Input: dimensioned drawing with shaded views. Units: mm. Origin: part minimum x, y, z. A direction names the side the tool comes from. Give positions to 0.01 mm unless a question says otherwise; leave off trailing zeros. Order: outer loops, then holes, each group sorted by start corner. A loop starts at its lowest first (then second) coordinate and runs counter-clockwise, first axis right, second up. Notation, with made-up numbers: (11.5, 33.5) - (18.5, 33.5) arc R19 cw to (18.5, 42.5) - close; hole circle Ø8 at (-37, 64.5). An arc over 180 degrees is marked (long way). Use a Markdown table: item, result.
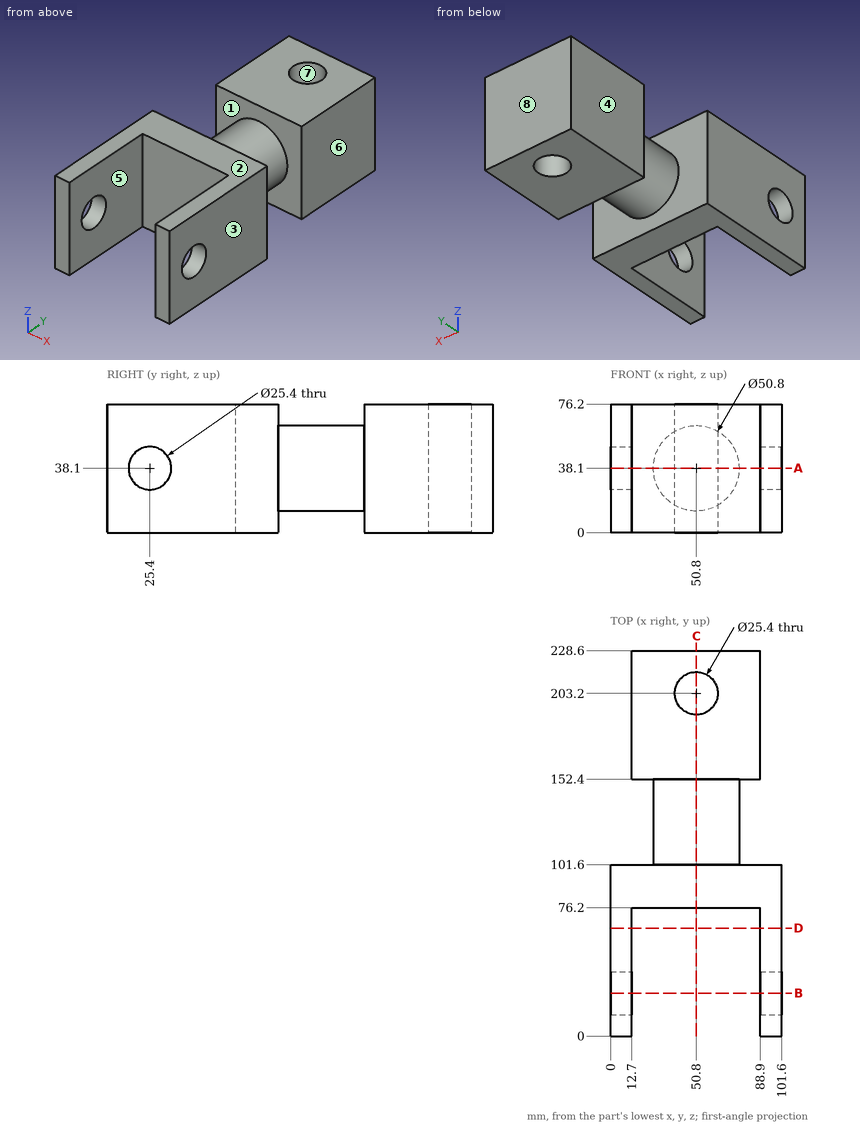
1. Mould query, pull axis X, two halves, no side actions, for the marked faces 6, 7 and 8. Classes: pulls with the +X half, pulls with the -X half, needs draft (parallel to the pull), parting line crosses it, or undercut.
Response:
| item | result |
|---|---|
| face 6 | pulls with the +X half |
| face 7 | undercut |
| face 8 | needs draft |
2. Pin query (flat end, axial travel): pin 1 (5 mm diameter, centred on y = 189.5, z = 42, fed in from -X); pin 2 (4 mm diameter, centred on x = 78.5, z = 17, fed in from -Y); pin 3 (1 mm diameter, centred on y = 176.5, z = 63, fed in from +X). Return the tip coordinate at first contact, or that it passes through.
Response:
| item | result |
|---|---|
| pin 1 | stops at x = 12.7 |
| pin 2 | stops at y = 76.2 |
| pin 3 | stops at x = 88.9 |
3. Section query C-C (x = 50.8). Return loops of the section in (y, z), then the cut area to 3 significant figures.
Response:
| item | result |
|---|---|
| outline | (76.2, 0) - (101.6, 0) - (101.6, 12.7) - (152.4, 12.7) - (152.4, 0) - (190.5, 0) - (190.5, 76.2) - (152.4, 76.2) - (152.4, 63.5) - (101.6, 63.5) - (101.6, 76.2) - (76.2, 76.2) - close; (215.9, 0) - (228.6, 0) - (228.6, 76.2) - (215.9, 76.2) - close |
| area | 8,390 mm^2 |
4. Set-up query: the marked faces 1, 2, 3, 4 and 5. Return all of +Z, -Z, +X, -X, +Y, -Y with unobstructed straight access to the full face (end or side cutting, diameter ignored); none if empty.
Response:
| item | result |
|---|---|
| face 1 | none |
| face 2 | +Z, +X, -X, +Y, -Y |
| face 3 | +Z, -Z, +X, +Y, -Y |
| face 4 | +Z, -Z, -X, +Y |
| face 5 | +Z, -Z, -Y |
5. Material intervals for line 1 along Y through (x, z) = (74.5, 15.5); line 2 along X through (y, z) = (21, 4); line 3 along Y through (x, z) = (50.8, 60), sorted ascending.
Response:
| item | result |
|---|---|
| line 1 | y = 76.2 to 101.6, 152.4 to 228.6 |
| line 2 | x = 0 to 12.7, 88.9 to 101.6 |
| line 3 | y = 76.2 to 190.5, 215.9 to 228.6 |
6. Section query A-A (z = 38.1). Return loops of the section in (x, y).
Response:
| item | result |
|---|---|
| outline | (0, 0) - (12.7, 0) - (12.7, 12.7) - (0, 12.7) - close; (0, 38.1) - (12.7, 38.1) - (12.7, 76.2) - (88.9, 76.2) - (88.9, 38.1) - (101.6, 38.1) - (101.6, 101.6) - (76.2, 101.6) - (76.2, 152.4) - (88.9, 152.4) - (88.9, 228.6) - (12.7, 228.6) - (12.7, 152.4) - (25.4, 152.4) - (25.4, 101.6) - (0, 101.6) - close; (88.9, 0) - (101.6, 0) - (101.6, 12.7) - (88.9, 12.7) - close; hole circle Ø25.4 at (50.8, 203.2) |
7. Section query B-B (y = 25.4). Return loops of the section in (x, z).
Response:
| item | result |
|---|---|
| outline | (0, 0) - (12.7, 0) - (12.7, 25.4) - (0, 25.4) - close; (0, 50.8) - (12.7, 50.8) - (12.7, 76.2) - (0, 76.2) - close; (88.9, 0) - (101.6, 0) - (101.6, 25.4) - (88.9, 25.4) - close; (88.9, 50.8) - (101.6, 50.8) - (101.6, 76.2) - (88.9, 76.2) - close |
8. Section query D-D (y = 64). Return loops of the section in (x, z), then the cut area to 3 significant figures.
Response:
| item | result |
|---|---|
| outline | (0, 0) - (12.7, 0) - (12.7, 76.2) - (0, 76.2) - close; (88.9, 0) - (101.6, 0) - (101.6, 76.2) - (88.9, 76.2) - close |
| area | 1,940 mm^2 |
